Geometry: final body of the model. Coordinates: model frame, mm. A direction names the side the tool comes from. Give positions to 0.01 mm unless a question says otherwise; leave off trailing zeros. Loops run counter-clockwise (first coordinate to the right, second up) from the corner with the lowest first, then second, coordinate; pieces in that order, holes last. Notation, with made-up numbers: (46, 53) - (62, 53) arc R21 ccw to (62, 66) - close; hole circle Ø5 at (31.5, 14.25). An arc over 180 degrees is marked (long way). Answer in a Markdown table with one row per item.
from build123d import *

# Parameters (mm, degrees)
SKETCH_1_W                  = 22.9
SKETCH_1_H                  = 37.9
EXTRUDE_1_DEPTH             = 4
HOLE_WIZARD_M4_1_AT_2_COUNT = 2
HOLE_WIZARD_M4_1_AT_2_PITCH = 14.9
SKETCH_6_W                  = 17.9
SKETCH_6_H                  = 25.9
CUT_EXTRUDE_1_DEPTH         = 19
SKETCH_7_W                  = 7.9
SKETCH_7_H                  = 32.9
CUT_EXTRUDE_2_DEPTH         = 19
FILLET_1_R                  = 1.5
FILLET_2_R                  = 1.5


with BuildPart() as part:
    # 草图1 → 凸台-拉伸1 (new, symmetric)
    with BuildSketch(Plane.XY):
        Rectangle(SKETCH_1_W, SKETCH_1_H)
    extrude(amount=EXTRUDE_1_DEPTH, both=True)

    # 草图5 → M4 螺纹孔1 (revolve, cut)
    with BuildSketch(Plane(origin=(-7.45, 18.95, 0), x_dir=(0, 0, 1), z_dir=(1, 0, 0))):
        Polygon((0, 0), (0, 9.091420021), (1.65, 8.1), (1.65, 0), align=None)
    hole_wizard_m4_1 = revolve(axis=Axis((-7.45, 25.3, 0), (0, -1, 0)), mode=Mode.SUBTRACT)

    # M4 螺纹孔1 at 2: M4 螺纹孔1 ×2
    with Locations(*[(i * HOLE_WIZARD_M4_1_AT_2_PITCH, 0, 0) for i in range(1, HOLE_WIZARD_M4_1_AT_2_COUNT)]):
        add(hole_wizard_m4_1, mode=Mode.SUBTRACT)

    # 镜向1: M4 螺纹孔1 across plane
    add(hole_wizard_m4_1.mirror(Plane.ZX), mode=Mode.SUBTRACT)

    # 镜向1 copy 1 sketch → 镜向1 copy 1 (revolve, cut)
    with BuildSketch(Plane(origin=(7.45, -18.95, 0), x_dir=(0, 0, 1), z_dir=(1, 0, 0))):
        Polygon((0, 0), (0, -9.091420021), (1.65, -8.1), (1.65, 0), align=None)
    revolve(axis=Axis((7.45, -25.3, 0), (0, -1, 0)), mode=Mode.SUBTRACT)

    # 草图6 → 切除-拉伸1 (cut, symmetric)
    with BuildSketch(Plane.XY.offset(4)):
        Rectangle(SKETCH_6_W, SKETCH_6_H)
    extrude(amount=CUT_EXTRUDE_1_DEPTH, both=True, mode=Mode.SUBTRACT)

    # 草图7 → 切除-拉伸2 (cut, symmetric)
    with BuildSketch(Plane.XY.offset(4)):
        Rectangle(SKETCH_7_W, SKETCH_7_H)
    extrude(amount=CUT_EXTRUDE_2_DEPTH, both=True, mode=Mode.SUBTRACT)

    # 圆角1
    fillet_1_edges = [part.edges().sort_by_distance(p)[0] for p in [
        (-8.95, 12.95, 2.343693177),
        (-8.95, 12.95, -2.343693177),
        (8.95, 12.95, 2.343693177),
        (8.95, 12.95, -2.343693177),
        (8.95, -12.95, 2.343693177),
        (8.95, -12.95, -2.343693177),
        (-8.95, -12.95, 2.343693177),
        (-8.95, -12.95, -2.343693177),
        (-3.95, -12.95, 0),
        (3.95, -12.95, 0),
        (3.95, -16.45, 0),
        (-3.95, 16.45, 0),
        (3.95, 16.45, 0),
        (3.95, 12.95, 0),
        (-3.95, 12.95, 0),
        (-3.95, -16.45, 0),
    ]]
    fillet(fillet_1_edges, radius=FILLET_1_R)

    # 圆角2
    fillet_2_edges = [part.edges().sort_by_distance(p)[0] for p in [
        (11.45, -18.95, 0),
        (-11.45, -18.95, 0),
        (-11.45, 18.95, 0),
        (11.45, 18.95, 0),
    ]]
    fillet(fillet_2_edges, radius=FILLET_2_R)


solid = part.part
Q1. Cut plane A-A (y = -3). Output: boundary loops of the cut face in (x, z), and give its area (3 significant figures).
Check values:
| item | result |
|---|---|
| outline | (-11.45, -4) - (-8.95, -4) - (-8.95, 4) - (-11.45, 4) - close; (8.95, -4) - (11.45, -4) - (11.45, 4) - (8.95, 4) - close |
| area | 40.0 mm² |
Q2. First-contact query: pin 1 (4 mm diameter, centred on x = 7.45, z = 0, fed in from -Y); pin 2 (5 mm diameter, centred on x = -1.5, y = -10, fed in from +Z). Flat tips, straight axial feed; report the tip coordinate or a pass-through.
Check values:
| item | result |
|---|---|
| pin 1 | y = -18.95 |
| pin 2 | through |
Q3. Reachability of faces 1 (the flat face through (0, 18.95, 0)), 2 (the flat face through (5.8, -12.95, 0.9)), 3 (the cylindrical face through (9.06, -15.86, -0.36)) from +Z, -Z, +X, -X, +Y, -Y: full face, straight path, thin tool, end or side. Return the list, or none.
Check values:
| item | result |
|---|---|
| face 1 | +Z, -Z, +X, -X, +Y |
| face 2 | +Z, -Z |
| face 3 | -Y |
Q4. Material intervals for line 1 along X through (y, z) = (17.25, 0); line 2 along X through (y, z) = (-2, 2.75); line 3 along Z through (x, y) = (-7.45, 14.5), sorted ascending.
Check values:
| item | result |
|---|---|
| line 1 | -11.45 to -9.1, -5.8 to 5.8, 9.1 to 11.45 |
| line 2 | -11.45 to -8.95, 8.95 to 11.45 |
| line 3 | -4 to -1.65, 1.65 to 4 |
Q5. Cut plane C-C (z = 0). Give the number of separate pieces and of enclosed holes in the cut face, and give its area (3 significant figures).
Check values:
| item | result |
|---|---|
| separate pieces | 4 |
| enclosed holes | 0 |
| area | 267 mm² |
Q6. Draft query along Y for faces 4 (the cylindrical face through (-9.086, 15.857, -0.215)), 5 (the cylindrical face through (11, -18.52, 0.06)), 6 (the flat face through (0, -16.45, 0)). Return one class per face: pulls with the +Y half, pulls with the -Y half, needs draft (parallel to the pull), parting line crosses it, or undercut.
Check values:
| item | result |
|---|---|
| face 4 | needs draft |
| face 5 | pulls with the -Y half |
| face 6 | undercut |
